Answer from the drawing. Dimensions are ordinates in mm from the lowest x, y and z of the part. A direction names the side the tool comes from. Round coordinates to 2 decimals unless told otherwise and drop trailing zeros. Write each loop counter-clockwise with the first axis right and the second up, starting at its lowest first coordinate (ties: lowest second). Pieces come first, ordered by that corner, then holes. Notation, with made-up numbers: (37.25, -16) -> (50.25, -16) arc R22 ccw to (50.25, 18) -> close; hole circle Ø8 at (-2, 87). An arc over 180 degrees is marked (long way). Return JSON: item names as keys, results as strings. Group by question number.
(1) For the marked faces 4 and 5, determine the directions among +Z, -Z, +X, -X, +Y, -Y from which every point of the face is accessible in a straight line to the end or side of a thin tool.
(2) A cutting plane is placed at C-C on z = 18. Give the vertices of the cut face in (x, y) (1 decimal), then the cut area to 3 significant figures.
(3) Straight lines are drawn through the part: line 1 (Z direction, x = 2.54, y = 1.7); line 2 (Z direction, x = 23, y = 5); line 3 (X direction, y = 7.5, z = 24.5) (1 decimal). For each, find the intervals that lie inside material, in ascending order.
(4) Given pin 1 (2 mm diameter, centred on x = 25.04, z = 37.15, fed in from +Y); pin 2 (3 mm diameter, centred on y = 6.5, z = 21, fed in from +X) (1 decimal); pin 3 (1.8 mm diameter, centred on y = 6.5, z = 19, fed in from -X), each flat-ended and moving along its own axis, determine where each tip first touches the part or whether it passes through.
(5) A cutting plane is placed at B-B on x = 34. Give the vertices of the cut face in (y, z).
(6) A cutting plane is placed at A-A on y = 3.75. Give the vertices of the cut face in (x, z) (1 decimal).
(7) The mould has two halves that part along X. Classify the marked faces 1, 2 and 3: released by +X, released by -X, zero draft, split by the parting line, or undercut.
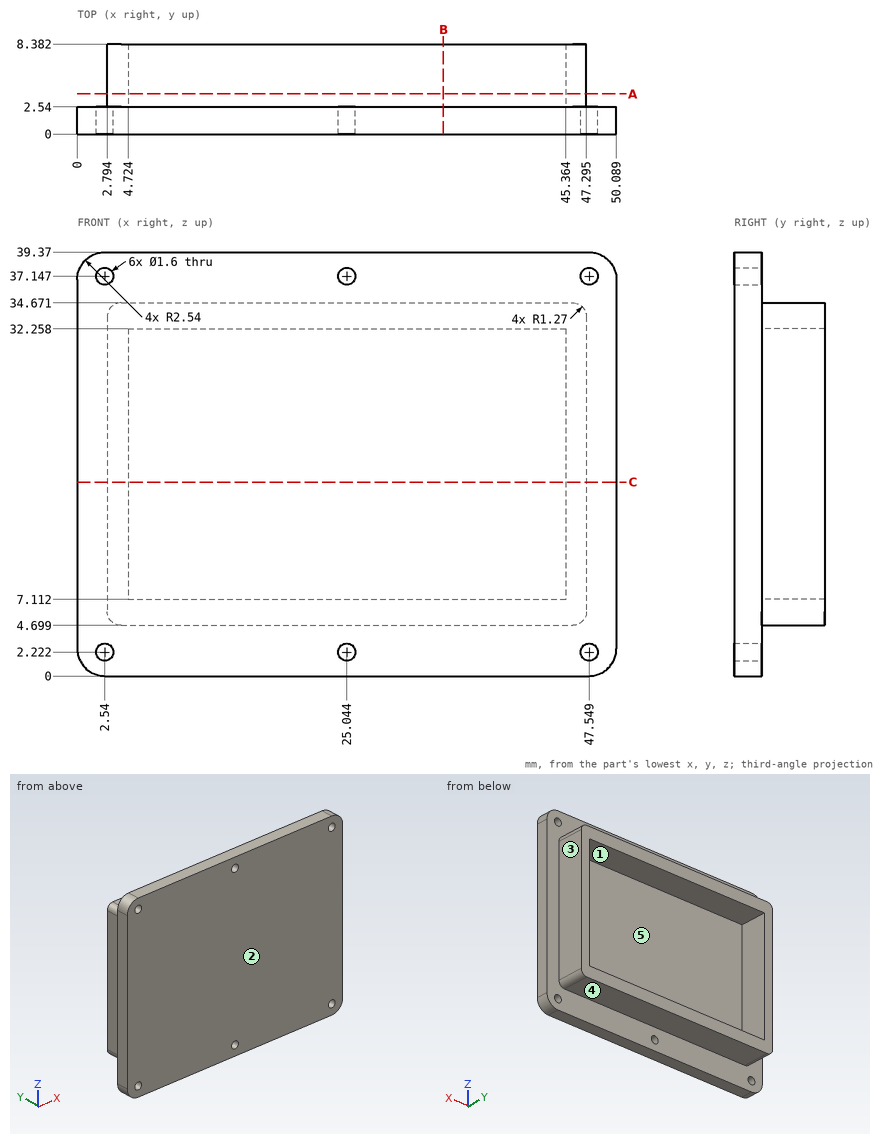
Checks:
{
 "1": {"face 4": "-Z, +X, -X, +Y", "face 5": "+Y"},
 "2": {"outline": "(0, 0) -> (50.1, 0) -> (50.1, 2.5) -> (47.3, 2.5) -> (47.3, 8.4) -> (45.4, 8.4) -> (45.4, 2.5) -> (4.7, 2.5) -> (4.7, 8.4) -> (2.8, 8.4) -> (2.8, 2.5) -> (0, 2.5) -> close", "area": "150 mm^2"},
 "3": {"line 1": "z = 0 to 1.42, 3.02 to 36.35, 37.95 to 39.37", "line 2": "z = 4.7 to 7.11, 32.26 to 34.67", "line 3": "x = 2.8 to 4.7, 45.4 to 47.3"},
 "4": {"pin 1": "stops at y = 2.54", "pin 2": "stops at x = 47.3", "pin 3": "stops at x = 2.79"},
 "5": {"outline": "(0, 0) -> (2.54, 0) -> (2.54, 4.7) -> (8.38, 4.7) -> (8.38, 7.11) -> (2.54, 7.11) -> (2.54, 32.26) -> (8.38, 32.26) -> (8.38, 34.67) -> (2.54, 34.67) -> (2.54, 39.37) -> (0, 39.37) -> close"},
 "6": {"outline": "(2.8, 6) arc R1.3 ccw to (4.1, 4.7) -> (46, 4.7) arc R1.3 ccw to (47.3, 6) -> (47.3, 33.4) arc R1.3 ccw to (46, 34.7) -> (4.1, 34.7) arc R1.3 ccw to (2.8, 33.4) -> close; hole (4.7, 7.1) -> (45.4, 7.1) -> (45.4, 32.3) -> (4.7, 32.3) -> close"},
 "7": {"face 1": "undercut", "face 2": "zero draft", "face 3": "released by +X"}
}
